The model under review builds one solid part; all positions refer to its coordinate system, in mm. Face numbers are marked on the shaded views. A direction names the side the tool comes from. Give positions to 0.01 mm unless a question says otherwise; leave off trailing zeros. Order: outer loops, then holes, each group sorted by start corner. A loop starts at its lowest first (then second) coordinate and runs counter-clockwise, first axis right, second up. Notation, with made-up numbers: (62.25, 7) - (114.25, 7) arc R16 ccw to (114.25, 21) - close; hole circle Ø9 at (40, 52). An arc over 180 degrees is marked (long way). Put each result on its own line as item: value.
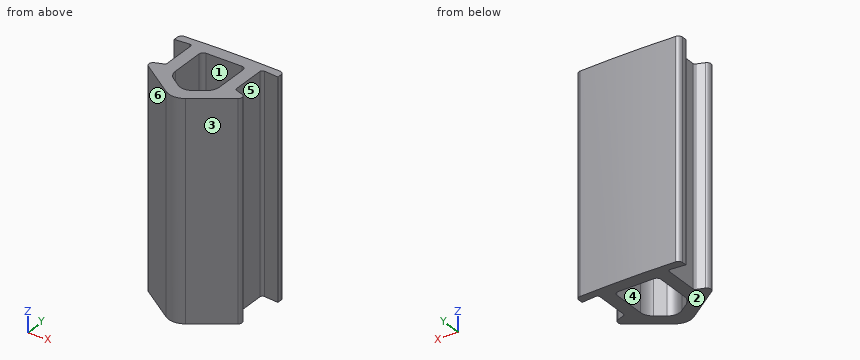
```python
from build123d import *

# Parameters (mm, degrees)
EXTRUSION4_DEPTH = 25.4


with BuildPart() as part:
    # Sketch1 → Extrusion4 (new body)
    with BuildSketch(Plane.XY):
        with BuildLine():
            ThreePointArc((5.643340731, 1.02471553), (5e-09, 1.14270907), (-5.643340721, 1.02471553))
            ThreePointArc((-5.643340721, 1.02471553), (-5.983308169, 0.871238001), (-6.12244139, 0.525152514))
            Line((-6.12244139, 0.525152514), (-6.12244139, 0))
            Line((-6.12244139, 0), (-4.426152829, 0.148406019))
            ThreePointArc((-4.426152829, 0.148406019), (-4.197329039, 0.070730809), (-4.1000061, -0.150452395))
            Line((-4.1000061, -0.150452395), (-4.1000061, -4.055821252))
            ThreePointArc((-4.1000061, -4.055821252), (-4.154260478, -4.227894187), (-4.297400051, -4.337729045))
            Line((-4.297400051, -4.337729045), (-5.171010065, -4.655697092))
            ThreePointArc((-5.171010065, -4.655697092), (-5.495722421, -5.060280306), (-5.286788207, -5.535119422))
            Line((-5.286788207, -5.535119422), (-1.147152857, -8.433723282))
            ThreePointArc((-1.147152857, -8.433723282), (1e-08, -8.79541919), (1.147152877, -8.433723282))
            Line((1.147152877, -8.433723282), (5.286788227, -5.535119422))
            ThreePointArc((5.286788227, -5.535119422), (5.495722441, -5.060280306), (5.171010085, -4.655697092))
            Line((5.171010085, -4.655697092), (4.297400071, -4.337729045))
            ThreePointArc((4.297400071, -4.337729045), (4.154260498, -4.227894187), (4.10000611, -4.055821252))
            Line((4.10000611, -4.055821252), (4.10000611, -0.15045238))
            ThreePointArc((4.10000611, -0.15045238), (4.197329045, 0.070730814), (4.426152823, 0.148406021))
            Line((4.426152823, 0.148406021), (6.1224414, 0))
            Line((6.1224414, 0), (6.1224414, 0.525152514))
            ThreePointArc((6.1224414, 0.525152514), (5.983308179, 0.871238001), (5.643340731, 1.02471553))
        make_face()
        with BuildLine():
            ThreePointArc((-2.100006108, -0.35045215), (-2.4535595, -0.49689876), (-2.60000611, -0.850452152))
            Line((-2.60000611, -0.850452152), (-2.60000611, -4.804412051))
            ThreePointArc((-2.60000611, -4.804412051), (-2.430522356, -5.497034977), (-1.960370752, -6.033140126))
            Line((-1.960370752, -6.033140126), (-0.860364633, -6.803372685))
            ThreePointArc((-0.860364633, -6.803372685), (2e-08, -7.07464461), (0.860364668, -6.803372674))
            Line((0.860364668, -6.803372674), (1.960370758, -6.033140115))
            ThreePointArc((1.960370758, -6.033140115), (2.430522351, -5.497034969), (2.6000061, -4.804412051))
            Line((2.6000061, -4.804412051), (2.6000061, -0.850452152))
            ThreePointArc((2.6000061, -0.850452152), (2.45355949, -0.49689876), (2.100006098, -0.35045215))
            Line((2.100006098, -0.35045215), (-2.100006108, -0.35045215))
        make_face(mode=Mode.SUBTRACT)
    extrude(amount=EXTRUSION4_DEPTH)


solid = part.part
```
(1) Take a section at C-C, the plane x = 1.5. Write out the cut boundary in (y, z), then the cut area to 3 significant figures.
The answers:
outline: (-8.19, 0) - (-6.36, 0) - (-6.36, 25.4) - (-8.19, 25.4) - close; (-0.35, 0) - (1.13, 0) - (1.13, 25.4) - (-0.35, 25.4) - close
area: 84.2 mm^2
(2) For the marked faces 4, 5 and 6, list the 3-axis set-ups (+Z, -Z, +X, -X, +Y, -Y) from which the entire face can be reached by the end or side of a thin tool; tool diameter is ignored.
The answers:
face 4: +Z, -Z
face 5: +Z, -Z, +X
face 6: +Z, -Z, -X, -Y
(3) Wall thickness on L1, parallel to X at y = -1.5, z = 15; L2, parallel to X at y = -5.25, z = 3; L3, parallel to Y at x = -0.25, z = 24.25: over which ranges is each line inside the solid? List them lowest first.
The answers:
L1: -4.1 to -2.6, 2.6 to 4.1
L2: -5.48 to -2.53, 2.53 to 5.48
L3: -8.78 to -7.05, -0.35 to 1.14
(4) Take a section at D-D, the plane x = 3. Write out the cut boundary in (y, z), then the cut area to 3 significant figures.
The answers:
outline: (-7.14, 0) - (1.11, 0) - (1.11, 25.4) - (-7.14, 25.4) - close
area: 209 mm^2
(5) Take a section at A-A, the plane y = -3.5. Write out the cut boundary in (x, z).
The answers:
outline: (-4.1, 0) - (-2.6, 0) - (-2.6, 25.4) - (-4.1, 25.4) - close; (2.6, 0) - (4.1, 0) - (4.1, 25.4) - (2.6, 25.4) - close
(6) The part is to be moulded in two halves that separate along Y. For the marked faces 1, 2 and 3, say which applies: pulls with the +Y half, pulls with the -Y half, needs draft (parallel to the pull), parting line crosses it, or undercut.
The answers:
face 1: undercut
face 2: needs draft
face 3: pulls with the -Y half
(7) Clearance check with flat-ended pins moving along their axes: pin 1 Ø3 at (y, z) = (-2, 20.5) entering from +X; pin 2 Ø2 at (x, z) = (4.5, 11) entering from -Y; pin 3 Ø2 at (y, z) = (-2.5, 17) entering from -X. State where each tip first meets the part, or that it passes through.
The answers:
pin 1: x = 4.1
pin 2: y = -6.79
pin 3: x = -4.1
